```python
from build123d import *

# Parameters (mm, degrees)
SKETCH1_R                      = 2.25
BASE_FLANGE1_DEPTH             = 0.1
EDGE_FLANGE1_STRIP_W           = 0.6
EDGE_FLANGE1_STRIP_H           = 0.1
EDGE_FLANGE1_STRIP_CUT_DEPTH   = 10.83
EDGE_FLANGE1_STRIP_2_W         = 0.6
EDGE_FLANGE1_STRIP_2_H         = 0.1
EDGE_FLANGE1_STRIP_CUT_2_DEPTH = 10.83
EDGE_FLANGE1_DEPTH             = 10.83
EDGE_FLANGE1_BEND_DEPTH        = 10.83
EDGE_FLANGE2_STRIP_W           = 0.6
EDGE_FLANGE2_STRIP_H           = 0.1
EDGE_FLANGE2_STRIP_CUT_DEPTH   = 10.83
EDGE_FLANGE2_STRIP_2_W         = 0.6
EDGE_FLANGE2_STRIP_2_H         = 0.1
EDGE_FLANGE2_STRIP_CUT_2_DEPTH = 10.83
EDGE_FLANGE2_DEPTH             = 10.83
EDGE_FLANGE2_BEND_DEPTH        = 10.83
CUT_EXTRUDE1_DEPTH             = 13.595815176
CUT_EXTRUDE1_DEPTH_BACK        = 13.595815176
CUT_EXTRUDE2_START             = -2.6
CUT_EXTRUDE2_OUTLINE_W         = 3
CUT_EXTRUDE2_OUTLINE_H         = 0.2
CUT_EXTRUDE2_DEPTH             = 2.6
TAB1_DEPTH                     = 0.1
CUT_EXTRUDE3_REACH             = 14.596
SKETCH23_R                     = 0.75
CUT_EXTRUDE3_DIRECTION_2_DEPTH = 13.595815176
BREAK_CORNER1_START            = -6.5
BREAK_CORNER1_DEPTH            = 0.1
FILLET1_R                      = 0.3
SKETCH24_R                     = 0.25
CUT_EXTRUDE4_DEPTH             = 10


# Read off the part's stored shape, not the designer's step: Cut-Extrude2, Break-Corner1
# Sheet-metal steps are written as plain solids
with BuildPart() as part:
    # Sketch1 → Base-Flange1 (new body)
    with BuildSketch(Plane(origin=(0, 0, 0), x_dir=(1, 0, 0), z_dir=(0, 1, 0))):
        with BuildLine():
            Line((-8.665102996, -2.95), (2.164897004, -2.95))
            Line((2.164897004, -2.95), (2.164897004, -2.75))
            ThreePointArc((2.164897004, -2.75), (3.499897004, 0), (2.164897004, 2.75))
            Line((2.164897004, 2.75), (2.164897004, 2.95))
            Line((2.164897004, 2.95), (-8.665102996, 2.95))
            Line((-8.665102996, 2.95), (-8.665102996, 2.75))
            ThreePointArc((-8.665102996, 2.75), (-10.000102996, 0), (-8.665102996, -2.75))
            Line((-8.665102996, -2.75), (-8.665102996, -2.95))
        make_face()
        with Locations(Location((0, 0, 0), (0, 0, 270))):
            Circle(SKETCH1_R, mode=Mode.SUBTRACT)
        with Locations(Location((-6.500205993, 0, 0), (0, 0, 270))):
            Circle(SKETCH1_R, mode=Mode.SUBTRACT)
    extrude(amount=-BASE_FLANGE1_DEPTH)

    # Edge-Flange1 strip (across the edge) → Edge-Flange1 strip cut (cut)
    with BuildSketch(Plane(origin=(2.164897004, -0.1, 2.95), x_dir=(0, 0, -1), z_dir=(-1, 0, 0))):
        with Locations((-0.1, -0.05)):
            Rectangle(EDGE_FLANGE1_STRIP_W, EDGE_FLANGE1_STRIP_H)
    extrude(amount=EDGE_FLANGE1_STRIP_CUT_DEPTH, mode=Mode.SUBTRACT)

    # Edge-Flange1 strip 2 (across the edge) → Edge-Flange1 strip cut 2 (cut)
    with BuildSketch(Plane(origin=(-8.665102996, -0.1, -2.95), x_dir=(0, 0, 1), z_dir=(1, 0, 0))):
        with Locations((-0.1, -0.05)):
            Rectangle(EDGE_FLANGE1_STRIP_2_W, EDGE_FLANGE1_STRIP_2_H)
    extrude(amount=EDGE_FLANGE1_STRIP_CUT_2_DEPTH, mode=Mode.SUBTRACT)

    # Edge-Flange1 section (across the edge) → Edge-Flange1 (add)
    with BuildSketch(Plane(origin=(2.164897004, -0.1, 2.95), x_dir=(0, 0, -1), z_dir=(-1, 0, 0))):
        with BuildLine():
            Line((0, 0.1), (0, 6.4))
            Line((0, 6.4), (0.1, 6.4))
            Line((0.1, 6.4), (0.1, 0.1))
            ThreePointArc((0.1, 0.1), (0.129289322, 0.029289322), (0.2, 0))
            Line((0.2, 0), (0.2, -0.1))
            ThreePointArc((0.2, -0.1), (0.058578644, -0.041421356), (0, 0.1))
        make_face()
    extrude(amount=EDGE_FLANGE1_DEPTH)

    # Edge-Flange1 section 2 (across the edge) → Edge-Flange1 bend (add)
    with BuildSketch(Plane(origin=(-8.665102996, -0.1, -2.95), x_dir=(0, 0, 1), z_dir=(1, 0, 0))):
        with BuildLine():
            Line((0, 0.1), (0, 6.4))
            Line((0, 6.4), (0.1, 6.4))
            Line((0.1, 6.4), (0.1, 0.1))
            ThreePointArc((0.1, 0.1), (0.129289322, 0.029289322), (0.2, 0))
            Line((0.2, 0), (0.2, -0.1))
            ThreePointArc((0.2, -0.1), (0.058578644, -0.041421356), (0, 0.1))
        make_face()
    extrude(amount=EDGE_FLANGE1_BEND_DEPTH)

    # Edge-Flange2 strip (across the edge) → Edge-Flange2 strip cut (cut)
    with BuildSketch(Plane(origin=(-8.665102996, -6.5, 2.95), x_dir=(0, 1, 0), z_dir=(1, 0, 0))):
        with Locations((-0.1, -0.05)):
            Rectangle(EDGE_FLANGE2_STRIP_W, EDGE_FLANGE2_STRIP_H)
    extrude(amount=EDGE_FLANGE2_STRIP_CUT_DEPTH, mode=Mode.SUBTRACT)

    # Edge-Flange2 strip 2 (across the edge) → Edge-Flange2 strip cut 2 (cut)
    with BuildSketch(Plane(origin=(2.164897004, -6.5, -2.95), x_dir=(0, 1, 0), z_dir=(-1, 0, 0))):
        with Locations((-0.1, -0.05)):
            Rectangle(EDGE_FLANGE2_STRIP_2_W, EDGE_FLANGE2_STRIP_2_H)
    extrude(amount=EDGE_FLANGE2_STRIP_CUT_2_DEPTH, mode=Mode.SUBTRACT)

    # Edge-Flange2 section (across the edge) → Edge-Flange2 (add)
    with BuildSketch(Plane(origin=(-8.665102996, -6.5, 2.95), x_dir=(0, 1, 0), z_dir=(1, 0, 0))):
        with BuildLine():
            Line((0, 0.1), (0, 1.1))
            Line((0, 1.1), (0.1, 1.1))
            Line((0.1, 1.1), (0.1, 0.1))
            ThreePointArc((0.1, 0.1), (0.129289322, 0.029289322), (0.2, 0))
            Line((0.2, 0), (0.2, -0.1))
            ThreePointArc((0.2, -0.1), (0.058578644, -0.041421356), (0, 0.1))
        make_face()
    extrude(amount=EDGE_FLANGE2_DEPTH)

    # Edge-Flange2 section 2 (across the edge) → Edge-Flange2 bend (add)
    with BuildSketch(Plane(origin=(2.164897004, -6.5, -2.95), x_dir=(0, 1, 0), z_dir=(-1, 0, 0))):
        with BuildLine():
            Line((0, 0.1), (0, 1.1))
            Line((0, 1.1), (0.1, 1.1))
            Line((0.1, 1.1), (0.1, 0.1))
            ThreePointArc((0.1, 0.1), (0.129289322, 0.029289322), (0.2, 0))
            Line((0.2, 0), (0.2, -0.1))
            ThreePointArc((0.2, -0.1), (0.058578644, -0.041421356), (0, 0.1))
        make_face()
    extrude(amount=EDGE_FLANGE2_BEND_DEPTH)

    # Sketch18 → Cut-Extrude1 (cut, two sides: drawn at the far end of the back side and taken through both)
    with BuildSketch(Plane.XY.offset(-CUT_EXTRUDE1_DEPTH_BACK)):
        with BuildLine():
            Line((-4.500102996, -6.5), (-4.500102996, -5))
            ThreePointArc((-4.500102996, -5), (-3.250102996, -3.75), (-2.000102996, -5))
            Line((-2.000102996, -5), (-2.000102996, -6.5))
            Line((-2.000102996, -6.5), (-4.500102996, -6.5))
        make_face()
    extrude(amount=CUT_EXTRUDE1_DEPTH + CUT_EXTRUDE1_DEPTH_BACK, mode=Mode.SUBTRACT)

    # Cut-Extrude2 outline → Cut-Extrude2 (cut)
    with BuildSketch(Plane(origin=(0, 0, 0), x_dir=(1, 0, 0), z_dir=(0, 1, 0)).offset(CUT_EXTRUDE2_START)):
        with Locations((-3.250102996, 2.85)):
            Rectangle(CUT_EXTRUDE2_OUTLINE_W, CUT_EXTRUDE2_OUTLINE_H)
        with Locations((-3.250102996, -2.85)):
            Rectangle(CUT_EXTRUDE2_OUTLINE_W, CUT_EXTRUDE2_OUTLINE_H)
    extrude(amount=CUT_EXTRUDE2_DEPTH, mode=Mode.SUBTRACT)

    # Sketch20 → Tab1 (add)
    with BuildSketch(Plane(origin=(0, 0, 0), x_dir=(1, 0, 0), z_dir=(0, 1, 0))):
        Polygon((-4.650102996, -2.75), (-4.650102996, -2.95), (-4.250102996, -4.05), (-2.250102996, -4.05), (-1.850102996, -2.95), (-1.850102996, -2.75), align=None)
    tab1 = extrude(amount=-TAB1_DEPTH)

    # Sketch23 → Cut-Extrude3 (cut, up to next)
    with BuildSketch(Plane(origin=(0, 0, 0), x_dir=(1, 0, 0), z_dir=(0, 1, 0)), mode=Mode.PRIVATE) as cut_extrude3_sk1:
        with Locations(Location((-3.250102996, -2.8, 0), (0, 0, 90))):
            Circle(SKETCH23_R)
    cut_extrude3_tool1 = extrude(cut_extrude3_sk1.sketch, amount=-CUT_EXTRUDE3_REACH, mode=Mode.PRIVATE) & part.part
    cut_extrude3 = cut_extrude3_tool1.solids().sort_by_distance((-3.250103, 0, 2.8))[0]
    add(cut_extrude3, mode=Mode.SUBTRACT)

    # Sketch23 → Cut-Extrude3 direction 2 (cut)
    with BuildSketch(Plane(origin=(0, 0, 0), x_dir=(1, 0, 0), z_dir=(0, 1, 0))):
        with Locations(Location((-3.250102996, -2.8, 0), (0, 0, 90))):
            Circle(SKETCH23_R)
    cut_extrude3_direction_2 = extrude(amount=CUT_EXTRUDE3_DIRECTION_2_DEPTH, mode=Mode.SUBTRACT)

    # Mirror1: Tab1, Cut-Extrude3, Cut-Extrude3 direction 2 across plane
    add(tab1.mirror(Plane.XY))
    add(cut_extrude3.mirror(Plane.XY), mode=Mode.SUBTRACT)
    add(cut_extrude3_direction_2.mirror(Plane.XY), mode=Mode.SUBTRACT)

    # Break-Corner1 outline → Break-Corner1 (cut)
    with BuildSketch(Plane(origin=(0, 0, 0), x_dir=(1, 0, 0), z_dir=(0, 1, 0)).offset(BREAK_CORNER1_START)):
        Polygon((-2.000102996, -4.05), (-1.700102996, -4.05), (-2.000102996, -3.75), align=None)
        Polygon((2.164897004, -3.75), (1.864897004, -4.05), (2.164897004, -4.05), align=None)
        Polygon((-4.500102996, -4.05), (-4.500102996, -3.75), (-4.800102996, -4.05), align=None)
        Polygon((-8.665102996, -4.05), (-8.365102996, -4.05), (-8.665102996, -3.75), align=None)
        Polygon((-2.000102996, 4.05), (-2.000102996, 3.75), (-1.700102996, 4.05), align=None)
        Polygon((2.164897004, 4.05), (1.864897004, 4.05), (2.164897004, 3.75), align=None)
        Polygon((-4.500102996, 4.05), (-4.800102996, 4.05), (-4.500102996, 3.75), align=None)
        Polygon((-8.665102996, 3.75), (-8.365102996, 4.05), (-8.665102996, 4.05), align=None)
    extrude(amount=BREAK_CORNER1_DEPTH, mode=Mode.SUBTRACT)

    # Fillet1
    # the kernel refuses this fillet: 0.3 mm, written as the material it takes off along each edge
    with BuildSketch(Plane(origin=(0, 0, 0), x_dir=(0, 0, 1), z_dir=(-1, 0, 0))) as fillet1_piece_1:
        with BuildLine():
            CenterArc((2.473606798, -0.3), FILLET1_R, 90, 48.189685104)
            Line((2.25, -0.1), (2.245527864, -0.096))
            ThreePointArc((2.245527864, -0.096), (2.244, -0.05), (2.244, 0))
            Line((2.244, 0), (2.25, 0.006))
            Line((2.25, 0.006), (2.473606798, 0.006))
            Line((2.473606798, 0.006), (2.473606798, 0))
        make_face()
    revolve(axis=Axis((0, 0, 0), (0, 1, 0)), mode=Mode.SUBTRACT)
    with BuildSketch(Plane(origin=(-6.500205993, 0, 0), x_dir=(0, 0, 1), z_dir=(-1, 0, 0))) as fillet1_piece_2:
        with BuildLine():
            CenterArc((2.473606798, -0.3), FILLET1_R, 90, 48.189685104)
            Line((2.25, -0.1), (2.245527864, -0.096))
            ThreePointArc((2.245527864, -0.096), (2.244, -0.05), (2.244, 0))
            Line((2.244, 0), (2.25, 0.006))
            Line((2.25, 0.006), (2.473606798, 0.006))
            Line((2.473606798, 0.006), (2.473606798, 0))
        make_face()
    revolve(axis=Axis((-6.500205993, 0, 0), (0, 1, 0)), mode=Mode.SUBTRACT)

    # Sketch24 → Cut-Extrude4 (cut)
    with BuildSketch(Plane(origin=(0, -6.4, 0), x_dir=(1, 0, 0), z_dir=(0, 1, 0))):
        with Locations(Location((-6.375102996, 3.6, 0), (0, 0, 270))):
            Circle(SKETCH24_R)
        with Locations(Location((-0.125102996, 3.6, 0), (0, 0, 90))):
            Circle(SKETCH24_R)
        with Locations(Location((-0.125102996, -3.6, 0), (0, 0, 270))):
            Circle(SKETCH24_R)
        with Locations(Location((-6.375102996, -3.6, 0), (0, 0, 90))):
            Circle(SKETCH24_R)
    extrude(amount=-CUT_EXTRUDE4_DEPTH, mode=Mode.SUBTRACT)


solid = part.part
```
Input: part model. Units: mm. Frame: model coordinates. Coordinates: 2 decimals unless noted, no trailing zeros. Write each loop counter-clockwise with the first axis right and the second up, starting at its lowest first coordinate (ties: lowest second). Pieces come first, ordered by that corner, then holes.
1) Section D-D on y = -5.25. Output: boundary loops of the cut face in (x, z).
2) Pin query (flat end, axial travel): pin 1 Ø2 at (x, z) = (-0.5, -0.5) entering from -Y; pin 2 Ø1.1 at (y, z) = (-4, -3) entering from -X; pin 3 Ø2 at (x, y) = (-1.5, -4) entering from +Z; pin 4 Ø1 at (x, y) = (-6.5, -3) entering from -Z. Return the tip coordinate at first contact, or that it passes through.
3) Section A-A on y = -0.5. Output: boundary loops of the cut face in (x, z), and give its area (3 significant figures).
4) Section C-C on z = 1.5. State how many separate pieces and enclosed holes the cut face has, and give its area (3 significant figures).
5) Section B-B on y = -2.75. Output: boundary loops of the cut face in (x, z), and give its area (3 significant figures).
Check result:
1. outline: (-8.67, -2.95) - (-4.5, -2.95) - (-4.5, -2.85) - (-8.67, -2.85) - close; (-8.67, 2.85) - (-4.5, 2.85) - (-4.5, 2.95) - (-8.67, 2.95) - close; (-2, -2.95) - (2.16, -2.95) - (2.16, -2.85) - (-2, -2.85) - close; (-2, 2.85) - (2.16, 2.85) - (2.16, 2.95) - (-2, 2.95) - close
2. pin 1: passes through
2. pin 2: stops at x = -8.67
2. pin 3: stops at z = 2.95
2. pin 4: stops at z = -2.95
3. outline: (-8.67, -2.95) - (-4.75, -2.95) - (-4.75, -2.85) - (-8.67, -2.85) - close; (-8.67, 2.85) - (-4.75, 2.85) - (-4.75, 2.95) - (-8.67, 2.95) - close; (-1.75, -2.95) - (2.16, -2.95) - (2.16, -2.85) - (-1.75, -2.85) - close; (-1.75, 2.85) - (2.16, 2.85) - (2.16, 2.95) - (-1.75, 2.95) - close
3. area: 1.57 mm2
4. separate pieces: 3
4. enclosed holes: 0
4. area: 0.575 mm2
5. outline: (-8.67, -2.95) - (2.16, -2.95) - (2.16, -2.85) - (-8.67, -2.85) - close; (-8.67, 2.85) - (2.16, 2.85) - (2.16, 2.95) - (-8.67, 2.95) - close
5. area: 2.17 mm2
